Input: dimensioned drawing with shaded views. Units: mm. Origin: part minimum x, y, z. A direction names the side the tool comes from. Round coordinates to 2 decimals unless told otherwise and drop trailing zeros. Write each loop counter-clockwise with the first axis right and the second up, starting at its lowest first coordinate (ties: lowest second). Pieces come first, ordered by that corner, then holes. Notation, with made-up numbers: (-14, -19) -> (36, -19) arc R7 cw to (36, -11) -> close; hole circle Ø1 at (42, 11.5). An arc over 180 degrees is marked (long way). Return JSON: item names as keys, results as strings. Group by question number.
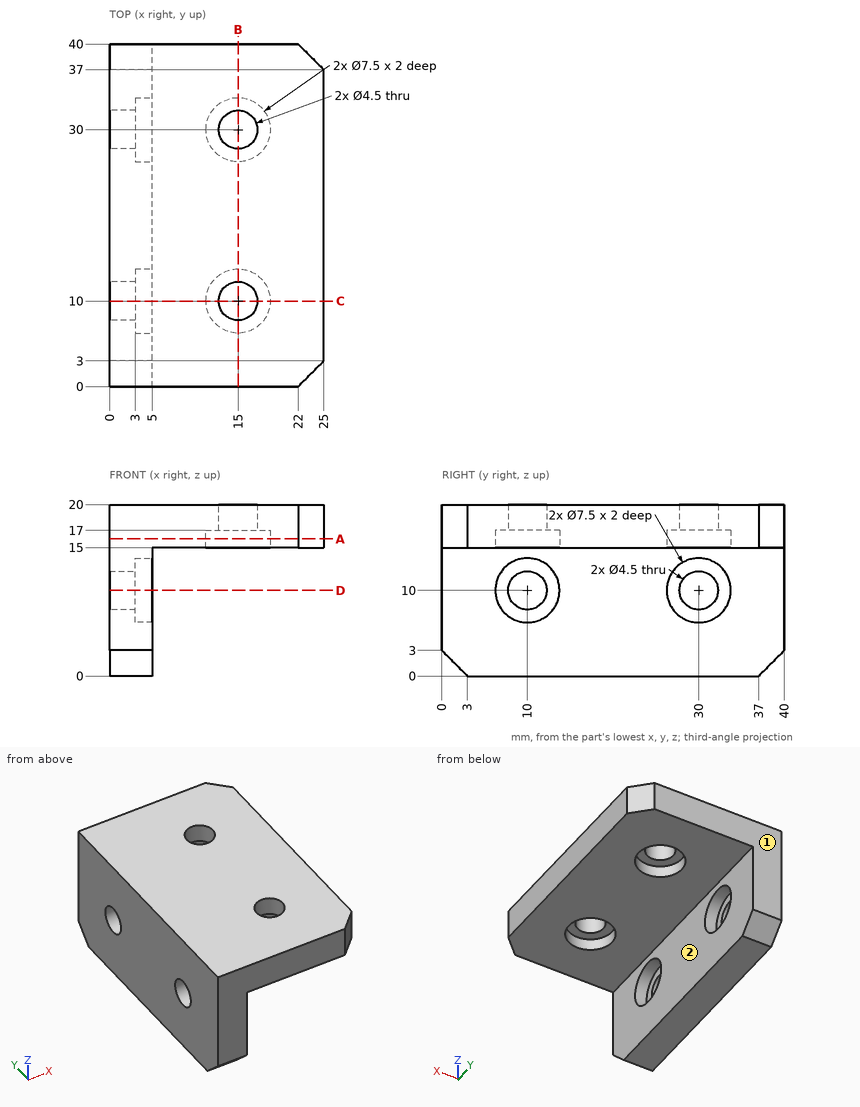
Item 1: Set-up query: the marked faces 1 and 2. Return all of +Z, -Z, +X, -X, +Y, -Y with unobstructed straight access to the full face (end or side cutting, diameter ignored); none if empty.
Item 2: Cut plane B-B on x = 15. Output: boundary loops of the cut face in (y, z).
Item 3: Material intervals for probe 1 along Y at (x, z) = (15, 15.75); probe 2 along Y at (x, z) = (1.4, 10); probe 3 along Z at (x, y) = (12, 20), sorted ascending.
Item 4: Cut plane C-C on y = 10. Output: boundary loops of the cut face in (x, z).
Item 5: Cut plane A-A on z = 16. Output: boundary loops of the cut face in (x, y).
Item 6: First-contact query: pin 1 Ø5 at (y, z) = (30, 10) entering from +X; pin 2 Ø3.5 at (y, z) = (10, 10) entering from +X; pin 3 Ø7 at (x, y) = (15, 10) entering from -Z; pin 4 Ø6 at (x, y) = (15.5, 11) entering from -Z. Flat tips, straight axial feed; report the tip coordinate or a pass-through.
Item 7: Cut plane D-D on z = 10. Output: boundary loops of the cut face in (x, y).
Here are the results:
{
 "1": {"face 1": "+Z, -Z, +X, -X, +Y", "face 2": "-Z, +X, +Y, -Y"},
 "2": {"outline": "(0, 15) -> (6.25, 15) -> (6.25, 17) -> (7.75, 17) -> (7.75, 20) -> (0, 20) -> close; (12.25, 17) -> (13.75, 17) -> (13.75, 15) -> (26.25, 15) -> (26.25, 17) -> (27.75, 17) -> (27.75, 20) -> (12.25, 20) -> close; (32.25, 17) -> (33.75, 17) -> (33.75, 15) -> (40, 15) -> (40, 20) -> (32.25, 20) -> close"},
 "3": {"probe 1": "y = 0 to 6.25, 13.75 to 26.25, 33.75 to 40", "probe 2": "y = 0 to 7.75, 12.25 to 27.75, 32.25 to 40", "probe 3": "z = 15 to 20"},
 "4": {"outline": "(0, 0) -> (5, 0) -> (5, 6.25) -> (3, 6.25) -> (3, 7.75) -> (0, 7.75) -> close; (0, 12.25) -> (3, 12.25) -> (3, 13.75) -> (5, 13.75) -> (5, 15) -> (11.25, 15) -> (11.25, 17) -> (12.75, 17) -> (12.75, 20) -> (0, 20) -> close; (17.25, 17) -> (18.75, 17) -> (18.75, 15) -> (25, 15) -> (25, 20) -> (17.25, 20) -> close"},
 "5": {"outline": "(0, 0) -> (22, 0) -> (25, 3) -> (25, 37) -> (22, 40) -> (0, 40) -> close; hole circle Ø7.5 at (15, 10); hole circle Ø7.5 at (15, 30)"},
 "6": {"pin 1": "stops at x = 3", "pin 2": "passes through", "pin 3": "stops at z = 17", "pin 4": "stops at z = 15"},
 "7": {"outline": "(0, 0) -> (5, 0) -> (5, 6.25) -> (3, 6.25) -> (3, 7.75) -> (0, 7.75) -> close; (0, 12.25) -> (3, 12.25) -> (3, 13.75) -> (5, 13.75) -> (5, 26.25) -> (3, 26.25) -> (3, 27.75) -> (0, 27.75) -> close; (0, 32.25) -> (3, 32.25) -> (3, 33.75) -> (5, 33.75) -> (5, 40) -> (0, 40) -> close"}
}
